Can you work these out from the drawing? Everything is in mm from the part's minimum corner. Coordinates: 2 decimals unless noted, no trailing zeros. Loops run counter-clockwise (first coordinate to the right, second up) from the corner with the lowest first, then second, coordinate; pieces in that order, holes last.
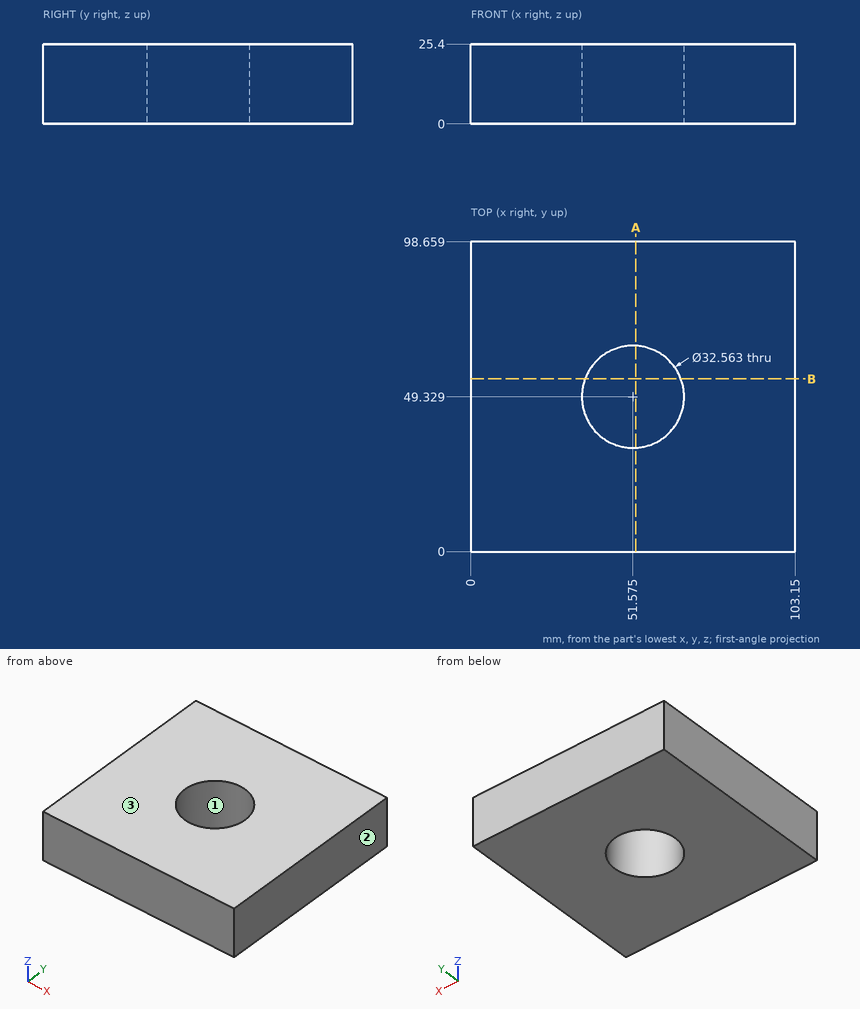
Item 1: We'd pull the mould along X, two halves only. Please class the marked faces 1, 2 and 3: +X half, -X half, draft (parallel to the pull), parting line (faces both ways), or undercut.
Results are:
face 1: undercut
face 2: +X half
face 3: draft
Item 2: Suppose I cut it at A-A, the plane x = 52.5. Please give me the cut outline in (y, z) (1 decimal).
Results are:
outline: (0, 0) - (33.1, 0) - (33.1, 25.4) - (0, 25.4) - close; (65.6, 0) - (98.7, 0) - (98.7, 25.4) - (65.6, 25.4) - close
Item 3: I need wall thicknesses on line 1 along X through (y, z) = (45, 4.25); line 2 along Y through (x, z) = (58, 3.5); line 3 along X through (y, z) = (38, 21). Which ranges of each line are inside material? Lowest first, please.
Results are:
line 1: x = 0 to 35.88, 67.27 to 103.15
line 2: y = 0 to 34.37, 64.29 to 98.66
line 3: x = 0 to 39.88, 63.27 to 103.15
Item 4: Suppose I cut it at B-B, the plane y = 55. Please give me the cut outline in (x, z), plus the area to 3 significant figures.
Results are:
outline: (0, 0) - (36.31, 0) - (36.31, 25.4) - (0, 25.4) - close; (66.84, 0) - (103.15, 0) - (103.15, 25.4) - (66.84, 25.4) - close
area: 1,840 mm2
